Check sheet for the modelled part. Datum: model origin and axes. Units: mm. A direction names the side the tool comes from. Round coordinates to 2 decimals unless told otherwise and drop trailing zeros. Order: outer loops, then holes, each group sorted by start corner. A loop starts at its lowest first (then second) coordinate and runs counter-clockwise, first axis right, second up. Notation, with made-up numbers: (1.25, -1) -> (36.25, -1) arc R19 cw to (36.25, 10) -> close; hole circle Ø1 at (52, 15.25). An arc over 180 degrees is marked (long way). Use CSV: the item, a comma, the result in double quotes.
```python
from build123d import *

# Parameters (mm, degrees)
SKETCH_1_R      = 5.25
SKETCH_1_R_2    = 3
EXTRUDE_1_DEPTH = 2
SKETCH_1_4_R    = 3
EXTRUDE_2_DEPTH = 27
FILLET_1_R      = 0.4
SKETCH_2_R      = 2.5
EXTRUDE_3_DEPTH = 0.9
SKETCH_3_R      = 3
EXTRUDE_4_DEPTH = 2.1
FILLET_2_R      = 0.4


with BuildPart() as part:
    # Sketch 1 → Extrude 1 (new body)
    with BuildSketch(Plane(origin=(0, 0, 0), x_dir=(0, 0, -1), z_dir=(1, 0, 0))):
        Circle(SKETCH_1_R)
        Circle(SKETCH_1_R_2, mode=Mode.SUBTRACT)
        Circle(SKETCH_1_R_2)
    extrude(amount=EXTRUDE_1_DEPTH)

    # Sketch 1_4 → Extrude 2 (add)
    with BuildSketch(Plane(origin=(0, 0, 0), x_dir=(0, 0, -1), z_dir=(1, 0, 0))):
        Circle(SKETCH_1_4_R)
    extrude(amount=-EXTRUDE_2_DEPTH)

    # Fillet 1
    fillet_1_edges = [part.edges().sort_by_distance(p)[0] for p in [
        (0, 0, 5.25),
        (2, 0, 5.25),
    ]]
    fillet(fillet_1_edges, radius=FILLET_1_R)

    # Sketch 2 → Extrude 3 (add)
    with BuildSketch(Plane.ZY.offset(27)):
        Circle(SKETCH_2_R)
    extrude(amount=EXTRUDE_3_DEPTH)

    # Sketch 3 → Extrude 4 (add)
    with BuildSketch(Plane.ZY.offset(27.9)):
        with Locations(Location((0, 0, 0), (0, 0, 180))):
            Circle(SKETCH_3_R)
    extrude(amount=EXTRUDE_4_DEPTH)

    # Fillet 2
    fillet_2_edges = [part.edges().sort_by_distance(p)[0] for p in [
        (-30, 0, 3),
    ]]
    fillet(fillet_2_edges, radius=FILLET_2_R)


solid = part.part
```
Q1. Scan lines: L1, parallel to X at y = -3.5, z = -1.25; L2, parallel to Z at x = -23, y = 1.5; L3, parallel to Z at x = -6.5, y = 2. Record each from-to range of solid material in increasing order.
Result sheet:
L1,"x = 0 to 2"
L2,"z = -2.6 to 2.6"
L3,"z = -2.24 to 2.24"
Q2. Mould release check, pull along X, two halves, no side actions. Record for faces 4 (the face through (0, 0.1, -3.2)), 5 (the face through (-27.9, -2, 2)), 6 (the face through (-13, 0, 3)), 7 (the face through (-27.44, -2.44, -0.54)): pulls with the +X half, pulls with the -X half, needs draft (parallel to the pull), parting line crosses it, or undercut.
Result sheet:
face 4,"pulls with the -X half"
face 5,"undercut"
face 6,"needs draft"
face 7,"undercut"
Q3. Access from +Z, -Z, +X, -X, +Y, -Y to the whole of each face (thin tool, end or side, straight path). Record for faces 1 (the face through (-28.74, -0.9, -2.86)), 2 (the face through (2, 0, 0)), 3 (the face through (-27, 2, 2)).
Result sheet:
face 1,"-X"
face 2,"+Z, -Z, +X, +Y, -Y"
face 3,"none"
Q4. Go/stop test with flat-tipped pins: pin 1 (3 mm diameter, centred on x = -5, z = 0, fed in from -Y); pin 2 (1 mm diameter, centred on x = -17, z = -2, fed in from -Y); pin 3 (4 mm diameter, centred on x = -24, z = 0, fed in from +Y). Record where each tip stops, or that it passes through.
Result sheet:
pin 1,"stops at y = -3"
pin 2,"stops at y = -2.6"
pin 3,"stops at y = 3"
Q5. Sectioned sample at C-C, the plane x = -11. Enter the section's corners in (y, z).
Result sheet:
outline,"circle Ø6 at (0, 0)"
Q6. Sectioned sample at A-A, the plane z = 0. Enter the section's corners in (x, y), then the cut area to 3 significant figures.
Result sheet:
outline,"(-30, -2.6) arc R0.4 ccw to (-29.6, -3) -> (-27.9, -3) -> (-27.9, -2.5) -> (-27, -2.5) -> (-27, -3) -> (0, -3) -> (0, -4.85) arc R0.4 ccw to (0.4, -5.25) -> (1.6, -5.25) arc R0.4 ccw to (2, -4.85) -> (2, 4.85) arc R0.4 ccw to (1.6, 5.25) -> (0.4, 5.25) arc R0.4 ccw to (0, 4.85) -> (0, 3) -> (-27, 3) -> (-27, 2.5) -> (-27.9, 2.5) -> (-27.9, 3) -> (-29.6, 3) arc R0.4 ccw to (-30, 2.6) -> close"
area,"200 mm^2"
